Verification items for the finished model (mm, model axes). Face numbers are marked on the shaded views. A direction names the side the tool comes from. Give positions to 0.01 mm unless a question says otherwise; leave off trailing zeros. Loops run counter-clockwise (first coordinate to the right, second up) from the corner with the lowest first, then second, coordinate; pieces in that order, holes last. Notation, with made-up numbers: (67, 47.5) - (115, 47.5) arc R17 cw to (115, 70.5) - close; hole circle Ø10 at (53.25, 54.25). An arc over 180 degrees is marked (long way). Put each result on its own line as item: value. Start each with the question number.
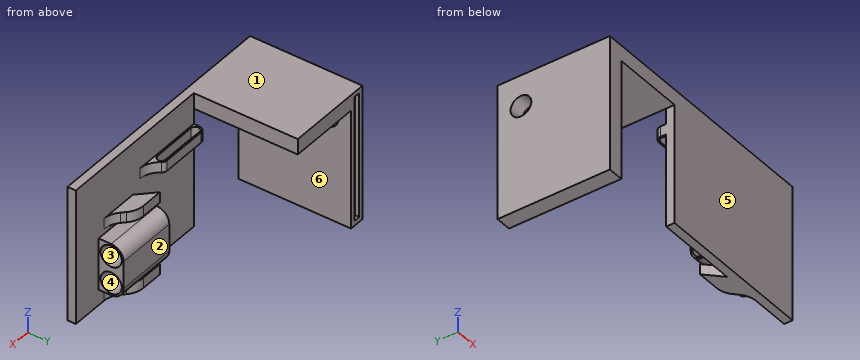
```python
from build123d import *

# Parameters (mm, degrees)
SKETCH1_W                       = 165
SKETCH1_H                       = 65
BOSS_EXTRUDE1_DEPTH             = 4
BOSS_EXTRUDE2_REACH             = 90.761
BOSS_EXTRUDE2_DIRECTION_2_DEPTH = 50
BOSS_EXTRUDE4_START             = -15
BOSS_EXTRUDE4_DEPTH             = 5
FILLET1_R                       = 10
BOSS_EXTRUDE5_DEPTH             = 5
FILLET3_R                       = 10
LPATTERN1_COUNT                 = 2
LPATTERN1_PITCH                 = 35
FILLET3_OF_LPATTERN1_R          = 10
SKETCH5_W                       = 82.5
SKETCH5_H                       = 65
CUT_EXTRUDE1_DEPTH              = 5
BOSS_EXTRUDE6_START             = -20
SKETCH6_R                       = 5.125000000000001
SKETCH6_R_2                     = 5.125
BOSS_EXTRUDE6_DEPTH             = 30
CUT_EXTRUDE6_DEPTH              = 2.1
SKETCH8_R                       = 4.999999999999999
CUT_EXTRUDE3_DEPTH              = 7.5
SKETCH19_W                      = 5
SKETCH19_H                      = 65
CUT_EXTRUDE11_DEPTH             = 10


with BuildPart() as part:
    # Sketch1 → Boss-Extrude1 (new body)
    with BuildSketch(Plane(origin=(0, 0, 0), x_dir=(1, 0, 0), z_dir=(0, 1, 0))):
        Rectangle(SKETCH1_W, SKETCH1_H)
    extrude(amount=BOSS_EXTRUDE1_DEPTH)

    # Boss-Extrude2: up to this face of the body (flat: up to its plane)
    boss_extrude2_end = Plane(part.part.faces().sort_by_distance((0, 0, 0))[0])
    # Sketch2 → Boss-Extrude2 (add, up to the picked face)
    with BuildSketch(Plane(origin=(0, 4, 0), x_dir=(1, 0, 0), z_dir=(0, 1, 0)), mode=Mode.PRIVATE) as boss_extrude2_sk1:
        Polygon((-82.5, -32.5), (-124.99999999999999, -32.50000000000001), (-124.99999999999999, 32.5), (-117.50000000000001, 32.5), (-117.50000000000001, -25), (-82.5, -25), align=None)
    boss_extrude2_tool1 = split(extrude(boss_extrude2_sk1.sketch, amount=-BOSS_EXTRUDE2_REACH, mode=Mode.PRIVATE), bisect_by=boss_extrude2_end, keep=Keep.BOTH, mode=Mode.PRIVATE)
    add(boss_extrude2_tool1.solids().sort_by(Axis((-103.75, 4, 31.723389), (0, -1, 0)))[0])

    # Sketch2 → Boss-Extrude2 direction 2 (add)
    with BuildSketch(Plane(origin=(0, 4, 0), x_dir=(1, 0, 0), z_dir=(0, 1, 0))):
        Polygon((-82.5, -32.5), (-124.99999999999999, -32.50000000000001), (-124.99999999999999, 32.5), (-117.50000000000001, 32.5), (-117.50000000000001, -25), (-82.5, -25), align=None)
    extrude(amount=BOSS_EXTRUDE2_DIRECTION_2_DEPTH)

    # Sketch3 → Boss-Extrude4 (add)
    with BuildSketch(Plane.XY.offset(32.5).offset(BOSS_EXTRUDE4_START)):
        with BuildLine():
            Line((-79.75, 9.500000000000004), (-57.50000000000001, 9.500000000000005))
            ThreePointArc((-57.50000000000001, 9.500000000000005), (-54.75000000000001, 6.75), (-57.50000000000001, 4))
            Line((-57.50000000000001, 4), (-82.5, 4))
            Line((-82.5, 4), (-82.5, 6.75))
            ThreePointArc((-82.5, 6.75), (-81.69454364826301, 8.694543648263005), (-79.75, 9.500000000000004))
        make_face()
        with BuildLine():
            Line((-79.75, 8.749999999999996), (-57.50000000000001, 8.75))
            ThreePointArc((-57.50000000000001, 8.75), (-55.50000000000001, 6.75), (-57.50000000000001, 4.749999999999999))
            Line((-57.50000000000001, 4.749999999999999), (-79.75, 4.750000000000004))
            ThreePointArc((-79.75, 4.750000000000004), (-81.75, 6.749999999999998), (-79.75, 8.749999999999996))
        make_face(mode=Mode.SUBTRACT)
    extrude(amount=-BOSS_EXTRUDE4_DEPTH)

    # Fillet1
    fillet1_edges = [part.edges().sort_by_distance(p)[0] for p in [
        (-57.50000000000001, 4.000000000000001, 15),
    ]]
    fillet(fillet1_edges, radius=FILLET1_R)

    # Sketch4 → Boss-Extrude5 (add)
    with BuildSketch(Plane(origin=(0, 0, -32.5), x_dir=(-1, 0, 0), z_dir=(0, 0, -1))):
        Polygon((27.500000000000004, 4), (35.00000000000008, 11.5), (50.00000000000008, 11.5), (42.5, 4), align=None)
    boss_extrude5 = extrude(amount=-BOSS_EXTRUDE5_DEPTH)

    # Fillet3
    fillet3_edges = [part.edges().sort_by_distance(p)[0] for p in [
        (-27.500000000000004, 4, -30),
        (-35.00000000000008, 11.5, -30),
    ]]
    fillet(fillet3_edges, radius=FILLET3_R)

    # LPattern1: Boss-Extrude5 ×2
    with Locations(*[(0, 0, i * LPATTERN1_PITCH) for i in range(1, LPATTERN1_COUNT)]):
        add(boss_extrude5)

    # Fillet3 of LPattern1
    fillet3_of_lpattern1_edges = [part.edges().sort_by_distance(p)[0] for p in [
        (-27.500000000000004, 4, 5),
        (-35.00000000000008, 11.5, 5),
    ]]
    fillet(fillet3_of_lpattern1_edges, radius=FILLET3_OF_LPATTERN1_R)

    # Sketch5 → Cut-Extrude1 (cut)
    with BuildSketch(Plane(origin=(0, 4, 0), x_dir=(1, 0, 0), z_dir=(0, 1, 0))):
        with Locations((41.25, 0)):
            Rectangle(SKETCH5_W, SKETCH5_H)
    extrude(amount=-CUT_EXTRUDE1_DEPTH, mode=Mode.SUBTRACT)

    # Sketch6 → Boss-Extrude6 (add)
    with BuildSketch(Plane(origin=(0, 0, 0), x_dir=(0, 0, -1), z_dir=(1, 0, 0)).offset(BOSS_EXTRUDE6_START)):
        with BuildLine():
            Line((1.1e-16, 10), (1.1e-16, 4))
            Line((1.1e-16, 4), (25, 4.0000000000000036))
            Line((25, 4.0000000000000036), (25, 10.000000000000002))
            ThreePointArc((25, 10.000000000000002), (23.242640687119287, 14.242640687119286), (19.000000000000004, 16))
            Line((19.000000000000004, 16), (6, 16))
            ThreePointArc((6, 16), (1.7573593128807152, 14.242640687119286), (1.1e-16, 10))
        make_face()
        with Locations((6.000000000000001, 10)):
            Circle(SKETCH6_R, mode=Mode.SUBTRACT)
        with Locations((19.000000000000004, 10.000000000000002)):
            Circle(SKETCH6_R_2, mode=Mode.SUBTRACT)
    extrude(amount=-BOSS_EXTRUDE6_DEPTH)

    # Sketch13 → Cut-Extrude6 (cut)
    with BuildSketch(Plane(origin=(0, 54.00000000000001, 0), x_dir=(1, 0, 0), z_dir=(0, 1, 0))):
        Polygon((-119.625, 30.15), (-122.875, 30.15), (-122.87499999999999, -30.150000000000006), (-119.625, -30.150000000000006), align=None)
    extrude(amount=-CUT_EXTRUDE6_DEPTH, mode=Mode.SUBTRACT)

    # Sketch8 → Cut-Extrude3 (cut)
    with BuildSketch(Plane.ZY.offset(124.99999999999999)):
        with Locations((17.50000000000002, 42.74019942711779)):
            Circle(SKETCH8_R)
    extrude(amount=-CUT_EXTRUDE3_DEPTH, mode=Mode.SUBTRACT)

    # Sketch19 → Cut-Extrude11 (cut)
    with BuildSketch(Plane(origin=(0, 4, 0), x_dir=(1, 0, 0), z_dir=(0, 1, 0))):
        with Locations((-2.5, 0)):
            Rectangle(SKETCH19_W, SKETCH19_H)
    extrude(amount=-CUT_EXTRUDE11_DEPTH, mode=Mode.SUBTRACT)


solid = part.part
```
1) Section check A-A, the plane x = -44.5. Enter the section's corners in (y, z) (3 decimals), plus the area to 3 significant figures.
2) Set-up check for the marked faces 4, 5 and 6: record each of +Z, -Z, +X, -X, +Y, -Y from which the full face is reachable in a straight line by a thin tool's end or side.
3) Section check C-C, the plane x = -74.5. Enter the section's corners in (y, z).
4) Depth check by flat-ended pin: P1, Ø2.5, axis at x = -44.5, z = -29, coming from the +Y side; P2, Ø5, axis at x = -63.5, y = 7, coming from the +Z side; P3, Ø6, axis at x = -33, y = 7.5, coming from the +Z side. Enter the tip coordinate at first touch or a pass-through.
5) Scan lines: line 1 along Y through (x, z) = (-31, -19) (3 decimals); line 2 along Y through (x, z) = (-22, 6.5); line 3 along Y through (x, z) = (-47.5, -1.5). Record each from-to range of solid material in increasing order. Write a range as from..to.
6) Draft check along Z on the marked faces 1, 2 and 3. Enter one of: pulls with the +Z half, pulls with the -Z half, needs draft (parallel to the pull), parting line crosses it, or undercut.
7) Section check D-D, the plane z = 21. Enter the section's corners in (x, y) (3 decimals).
8) Section check B-B, the plane y = 13.5. Enter the section's corners in (x, z).
Results are:
1. outline: (0, -32.5) - (4, -32.5) - (4, -25) - (10, -25) arc R6 ccw to (16, -19) - (16, -6) arc R6 ccw to (10, 0) - (4, 0) - (4, 32.5) - (0, 32.5) - close; (6, -32.5) - (11.5, -32.5) - (11.5, -27.5) - (6, -27.5) - close; (6, 2.5) - (11.5, 2.5) - (11.5, 7.5) - (6, 7.5) - close; hole circle Ø10.25 at (10, -19); hole circle Ø10.25 at (10, -6)
1. area: 435 mm2
2. face 4: +X
2. face 5: +Z, -Z, +X, -X, -Y
2. face 6: -Z, +Y, -Y
3. outline: (0, -32.5) - (4, -32.5) - (4, 12.5) - (4.75, 12.5) - (4.75, 17.5) - (4, 17.5) - (4, 32.5) - (0, 32.5) - close; (8.75, 12.5) - (9.5, 12.5) - (9.5, 17.5) - (8.75, 17.5) - close
4. P1: stops at y = 11.5
4. P2: stops at z = 17.5
4. P3: stops at z = 7.5
5. line 1: y = 0..4.875, 15.125..16
5. line 2: y = 0..4
5. line 3: y = 0..7.55, 12.45..13.97
6. face 1: pulls with the +Z half
6. face 2: needs draft
6. face 3: undercut
7. outline: (-125, 0) - (-117.5, 0) - (-117.5, 39.169) - (-125, 39.169) - close; (-125, 46.311) - (-117.5, 46.311) - (-117.5, 54) - (-119.625, 54) - (-119.625, 51.9) - (-122.875, 51.9) - (-122.875, 54) - (-125, 54) - close; (-82.5, 0) - (-5, 0) - (-5, 4) - (-82.5, 4) - close
8. outline: (-125, -32.5) - (-117.5, -32.5) - (-117.5, 25) - (-82.5, 25) - (-82.5, 32.5) - (-125, 32.5) - close; (-50, -23.87) - (-20, -23.87) - (-20, -22.74) - (-50, -22.74) - close; (-50, -15.26) - (-20, -15.26) - (-20, -9.74) - (-50, -9.74) - close; (-50, -2.26) - (-20, -2.26) - (-20, -1.13) - (-50, -1.13) - close
